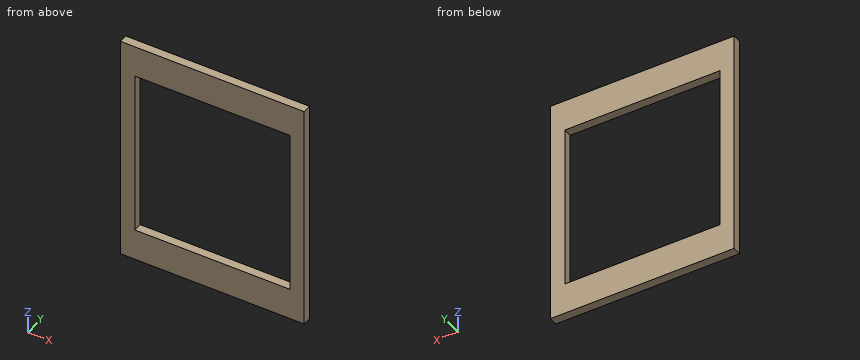
Autodesk Inventor part; units mm, degrees
ref_plane "YZ Plane" through (0, 0, 0) normal (1, 0, 0) x (0, 1, 0)
ref_plane "XZ Plane" through (0, 0, 0) normal (0, 1, 0) x (-1, 0, 0)
ref_plane "XY Plane" through (0, 0, 0) normal (0, 0, 1) x (1, 0, 0)
sketch "Sketch1" plane through (0, 0, 0) normal (0, 1, 0) x (-1, 0, 0)
  line L0 (-203.2, 254) -> (203.2, 254)
  line L1 (203.2, 254) -> (203.2, -254)
  line L2 (203.2, -254) -> (-203.2, -254)
  line L3 (-203.2, -254) -> (-203.2, 254)
  line L4 (-203.2, 254) -> (203.2, -254) construction
  line L5 (203.2, 254) -> (-203.2, -254) construction
  point P0 (0, 0)
  dimension "d0" = 508
  dimension "d1" = 406.4
extrude "Extrusion1" add sketch "Sketch1" along normal blind 19.05
sketch "Sketch2" plane through (0, 19.05, 0) normal (0, 1, 0) x (1, 0, 0)
  line L0 (171.45, -184.15) -> (-171.45, -184.15)
  line L1 (-171.45, -184.15) -> (-171.45, 184.15)
  line L2 (-171.45, 184.15) -> (171.45, 184.15)
  line L3 (171.45, 184.15) -> (171.45, -184.15)
  line L4 (171.45, -184.15) -> (-171.45, 184.15) construction
  line L5 (-171.45, -184.15) -> (171.45, 184.15) construction
  point P0 (0, 0)
  dimension "d4" = 368.3
  dimension "d5" = 342.9
extrude "Extrusion2" cut sketch "Sketch2" against normal blind 25.4
properties part number "monitor frame part1 (for assembly)"
Verification items for the finished model (mm, model axes). Give positions to 0.01 mm unless a question says otherwise; leave off trailing zeros. Loops run counter-clockwise (first coordinate to the right, second up) from the corner with the lowest first, then second, coordinate; pieces in that order, holes last. Notation, with made-up numbers: (40, 61.5) - (71, 61.5) arc R22 ccw to (71, 96.5) - close; hole circle Ø2 at (60.5, 72.5). An arc over 180 degrees is marked (long way). Write item = value, one per line. Start each with the question number.
Q1. Cross-section at C-C, the plane y = 11. Enter the section's corners in (x, z), and give its area (3 significant figures).
Q2. Cross-section at B-B, the plane x = -112.5. Enter the section's corners in (y, z).
Q3. Cross-section at A-A, the plane z = -173. Enter the section's corners in (x, y).
Q4. Thickness scan on line 1 (X direction, y = 10.75, z = 3.5); line 2 (Z direction, x = -83, y = 4). Record the ranges inside material, lowest first.
Answer key:
q1.outline = (-203.2, -254) - (203.2, -254) - (203.2, 254) - (-203.2, 254) - close; hole (-171.45, -184.15) - (171.45, -184.15) - (171.45, 184.15) - (-171.45, 184.15) - close
q1.area = 80,200 mm^2
q2.outline = (0, -254) - (19.05, -254) - (19.05, -184.15) - (0, -184.15) - close; (0, 184.15) - (19.05, 184.15) - (19.05, 254) - (0, 254) - close
q3.outline = (-203.2, 0) - (-171.45, 0) - (-171.45, 19.05) - (-203.2, 19.05) - close; (171.45, 0) - (203.2, 0) - (203.2, 19.05) - (171.45, 19.05) - close
q4.line_1 = -203.2 to -171.45, 171.45 to 203.2
q4.line_2 = -254 to -184.15, 184.15 to 254
